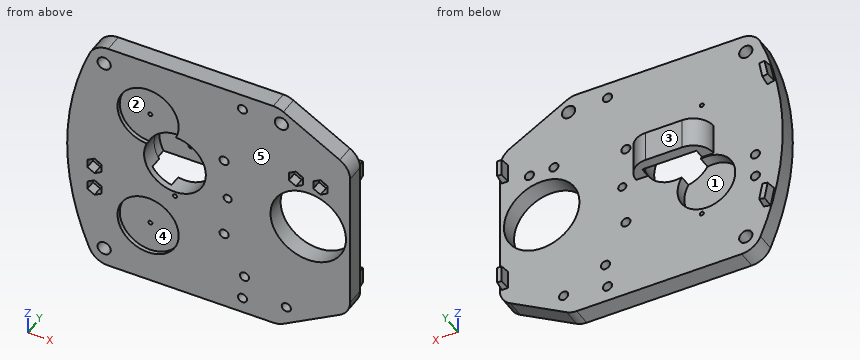
```python
from build123d import *

# Parameters (mm, degrees)
SKETCH1_W                         = 125
SKETCH1_H                         = 120
TOP_BASE_DEPTH                    = 9
SKETCH5_R                         = 14.15
DRIVE_GEAR_HOLE_DEPTH             = 6
SKETCH28_R                        = 15.15
TWO_STAGE_GEAR_HOLE_DEPTH         = 174.51080658
SKETCH8_R                         = 18.5
XL320_FINGER_KNUCKLE_MOUNT_DEPTH  = 174.51080658
SKETCH26_R                        = 1
STRING_HOLES_DEPTH                = 174.51080658
XL320_MOUNT_HOLES_R               = 2.25
XL320_MOUNT_HOLES_M4_DEPTH        = 174.51080658
AX12_MOUNT_HOLES_R                = 2.25
AX12_MOUNT_HOLES_M4_DEPTH         = 174.51080658
NUTS_M4_DEPTH                     = 5
SKETCH34_R                        = 15
HOLES_FOR_M4_IN_FINGER_GEAR_DEPTH = 2
SKETCH31_W                        = 38
SKETCH31_H                        = 15
BOSS_EXTRUDE1_DEPTH               = 10
SKETCH32_R                        = 15.25
CUT_EXTRUDE5_DEPTH                = 5
SKETCH33_R                        = 1
CUT_EXTRUDE6_DEPTH                = 2.5
FILLET2_R                         = 10
CUT_EXTRUDE8_DEPTH                = 174.565549577
FILLET4_R                         = 10
SKETCH37_R                        = 3.25
CONNECT_HOLES_M6_DEPTH            = 10
SKETCH41_R                        = 2
CONNECT_TO_HOUSE_M4_DEPTH         = 174.565549577
SKETCH42_W                        = 3
SKETCH42_H                        = 9
HOUSING_FITS_DEPTH                = 5
HOUSING_FITS_DRAFT                = 5
HOUSING_FITS_PROFILE_2_DEPTH      = 5
HOUSING_FITS_PROFILE_2_DRAFT      = 5
HOUSING_FITS_PROFILE_3_DEPTH      = 5
HOUSING_FITS_PROFILE_3_DRAFT      = 5
HOUSING_FITS_PROFILE_4_DEPTH      = 5
HOUSING_FITS_PROFILE_4_DRAFT      = 5
SKETCH43_R                        = 1
M2_SHAFT_HOLE_DEPTH               = 2


with BuildPart() as part:
    # Sketch1 → Top_Base (new body)
    with BuildSketch(Plane(origin=(0, 0, 0), x_dir=(1, 0, 0), z_dir=(0, 1, 0))):
        with BuildLine():
            ThreePointArc((0, 120), (-13.654246239, 60), (0, 0))
            Line((0, 0), (0, 120))
        make_face()
        with Locations((62.5, 60)):
            Rectangle(SKETCH1_W, SKETCH1_H)
    extrude(amount=TOP_BASE_DEPTH)

    # Sketch5 → Drive_Gear_Hole (cut)
    with BuildSketch(Plane(origin=(0, 9, 0), x_dir=(1, 0, 0), z_dir=(0, 1, 0))):
        with Locations(Location((23.75, 73.41386581, 0), (0, 0, 270))):
            Circle(SKETCH5_R)
    extrude(amount=-DRIVE_GEAR_HOLE_DEPTH, mode=Mode.SUBTRACT)

    # Sketch28 → Two_Stage_Gear_Hole (cut, through all)
    with BuildSketch(Plane(origin=(0, 9, 0), x_dir=(1, 0, 0), z_dir=(0, 1, 0))):
        with Locations(Location((39.169567191, 51.25, 0), (0, 0, 270))):
            Circle(SKETCH28_R)
    extrude(amount=-TWO_STAGE_GEAR_HOLE_DEPTH, mode=Mode.SUBTRACT)

    # Sketch8 → XL320_Finger_Knuckle_Mount (cut, through all)
    with BuildSketch(Plane(origin=(0, 9, 0), x_dir=(1, 0, 0), z_dir=(0, 1, 0))):
        with Locations(Location((104.5, 60, 0), (0, 0, 270))):
            Circle(SKETCH8_R)
    extrude(amount=-XL320_FINGER_KNUCKLE_MOUNT_DEPTH, mode=Mode.SUBTRACT)

    # Sketch26 → String_Holes (cut, through all)
    with BuildSketch(Plane.XZ.offset(-9)):
        with Locations(Location((26, -30, 0), (0, 0, 270))):
            Circle(SKETCH26_R)
        with Locations(Location((26, -90, 0), (0, 0, 90))):
            Circle(SKETCH26_R)
    extrude(amount=STRING_HOLES_DEPTH, mode=Mode.SUBTRACT)

    # XL320_Mount_Holes → XL320_Mount_Holes_(M4) (cut, through all)
    with BuildSketch(Plane(origin=(0, 9, 0), x_dir=(1, 0, 0), z_dir=(0, 1, 0))):
        with Locations(Location((110.5, 36, 0), (0, 0, 270))):
            Circle(XL320_MOUNT_HOLES_R)
        with Locations(Location((98.5, 36, 0), (0, 0, 270))):
            Circle(XL320_MOUNT_HOLES_R)
        with Locations(Location((-0.25, 79.41386581, 0), (0, 0, 270))):
            Circle(XL320_MOUNT_HOLES_R)
        with Locations(Location((-0.25, 67.41386581, 0), (0, 0, 270))):
            Circle(XL320_MOUNT_HOLES_R)
    extrude(amount=-XL320_MOUNT_HOLES_M4_DEPTH, mode=Mode.SUBTRACT)

    # AX12_Mount_Holes → AX12_Mount_Holes_(M4) (cut, through all)
    with BuildSketch(Plane(origin=(0, 9, 0), x_dir=(1, 0, 0), z_dir=(0, 1, 0))):
        with Locations(Location((72.25, 112.25, 0), (0, 0, 270))):
            Circle(AX12_MOUNT_HOLES_R)
        with Locations(Location((63.25, 80.25, 0), (0, 0, 270))):
            Circle(AX12_MOUNT_HOLES_R)
        with Locations(Location((73.25, 100, 0), (0, 0, 270))):
            Circle(AX12_MOUNT_HOLES_R)
        with Locations(Location((93.75, 109, 0), (0, 0, 270))):
            Circle(AX12_MOUNT_HOLES_R)
        with Locations(Location((63.25, 39.75, 0), (0, 0, 270))):
            Circle(AX12_MOUNT_HOLES_R)
        with Locations(Location((72.25, 7.75, 0), (0, 0, 270))):
            Circle(AX12_MOUNT_HOLES_R)
    extrude(amount=-AX12_MOUNT_HOLES_M4_DEPTH, mode=Mode.SUBTRACT)

    # Sketch27 → Nuts_(M4) (cut)
    with BuildSketch(Plane.XZ):
        Polygon((110.5, -31.958548116), (107, -33.979274058), (107, -38.020725942), (110.5, -40.041451884), (114, -38.020725942), (114, -33.979274058), align=None)
        Polygon((98.5, -31.958548116), (95, -33.979274058), (95, -38.020725942), (98.5, -40.041451884), (102, -38.020725942), (102, -33.979274058), align=None)
        Polygon((3.25, -65.393139868), (-0.25, -63.372413926), (-3.75, -65.393139868), (-3.75, -69.434591752), (-0.25, -71.455317694), (3.25, -69.434591752), align=None)
        Polygon((-3.75, -77.393139868), (-3.75, -81.434591752), (-0.25, -83.455317694), (3.25, -81.434591752), (3.25, -77.393139868), (-0.25, -75.372413926), align=None)
    extrude(amount=-NUTS_M4_DEPTH, mode=Mode.SUBTRACT)

    # Sketch34 → Holes_For_M4_In_Finger_Gear (cut)
    with BuildSketch(Plane.XZ):
        with Locations((26, -30)):
            Circle(SKETCH34_R)
        with Locations(Location((26, -90, 0), (0, 0, 270))):
            Circle(SKETCH34_R)
    extrude(amount=-HOLES_FOR_M4_IN_FINGER_GEAR_DEPTH, mode=Mode.SUBTRACT)

    # Sketch31 → Boss-Extrude1 (add)
    with BuildSketch(Plane(origin=(0, 9, 0), x_dir=(1, 0, 0), z_dir=(0, 1, 0))):
        with Locations((39.169567191, 51.25)):
            Rectangle(SKETCH31_W, SKETCH31_H)
    extrude(amount=BOSS_EXTRUDE1_DEPTH)

    # Sketch32 → Cut-Extrude5 (cut)
    with BuildSketch(Plane.XZ.offset(-9)):
        with Locations((39.169567191, -51.25)):
            Circle(SKETCH32_R)
    extrude(amount=-CUT_EXTRUDE5_DEPTH, mode=Mode.SUBTRACT)

    # Sketch33 → Cut-Extrude6 (cut)
    with BuildSketch(Plane.XZ.offset(-14)):
        with Locations(Location((39.169567191, -51.25, 0), (0, 0, 270))):
            Circle(SKETCH33_R)
    extrude(amount=-CUT_EXTRUDE6_DEPTH, mode=Mode.SUBTRACT)

    # Fillet2
    fillet2_edges = [part.edges().sort_by_distance(p)[0] for p in [
        (58.169567191, 19, -51.25),
        (20.169567191, 19, -51.25),
    ]]
    fillet(fillet2_edges, radius=FILLET2_R - 0.0001)  # a hair under: the kernel refuses the full size

    # Sketch36 → Cut-Extrude8 (cut, through all)
    with BuildSketch(Plane(origin=(0, 9, 0), x_dir=(1, 0, 0), z_dir=(0, 1, 0))):
        Polygon((90, 120), (125, 100), (125, 120), align=None)
        Polygon((125, 0), (90, 0), (125, 20), align=None)
    extrude(amount=-CUT_EXTRUDE8_DEPTH, mode=Mode.SUBTRACT)

    # Fillet4
    fillet4_edges = [part.edges().sort_by_distance(p)[0] for p in [
        (90, 4.5, -120),
        (125, 4.5, -100),
        (125, 4.5, -20),
        (90, 4.5, 0),
        (0, 4.5, -120),
        (0, 4.5, 0),
    ]]
    fillet(fillet4_edges, radius=FILLET4_R)

    # Sketch37 → Connect_Holes_(M6) (cut)
    with BuildSketch(Plane(origin=(0, 9, 0), x_dir=(1, 0, 0), z_dir=(0, 1, 0))):
        with Locations(Location((4.459226107, 111.152938298, 0), (0, 0, 270))):
            Circle(SKETCH37_R)
        with Locations(Location((4.459226107, 8.847061702, 0), (0, 0, 270))):
            Circle(SKETCH37_R)
        with Locations(Location((91.344355629, 8.205555711, 0), (0, 0, 270))):
            Circle(SKETCH37_R)
    extrude(amount=-CONNECT_HOLES_M6_DEPTH, mode=Mode.SUBTRACT)

    # Sketch41 → Connect_To_House_(M4) (cut, through all)
    with BuildSketch(Plane(origin=(0, 9, 0), x_dir=(1, 0, 0), z_dir=(0, 1, 0))):
        with Locations(Location((65, 60, 0), (0, 0, 270))):
            Circle(SKETCH41_R)
    extrude(amount=-CONNECT_TO_HOUSE_M4_DEPTH, mode=Mode.SUBTRACT)


with BuildPart() as housing_fits_tool:
    # Sketch42 → Housing_Fits (with draft: the straight prism first)
    with BuildSketch(Plane(origin=(0, 9, 0), x_dir=(1, 0, 0), z_dir=(0, 1, 0))):
        with Locations((122.5, 30.5)):
            Rectangle(SKETCH42_W, SKETCH42_H)
    extrude(amount=HOUSING_FITS_DEPTH)
    # Housing_Fits: the draft: its side faces are tilted about the plane it starts from
    housing_fits_sides = [housing_fits_tool.faces().sort_by_distance(p)[0] for p in [
        (124, 11.5, -30.5),
        (122.5, 11.5, -35),
        (121, 11.5, -30.5),
        (122.5, 11.5, -26),
    ]]
    draft(housing_fits_sides, Plane(origin=(0, 9, 0), x_dir=(1, 0, 0), z_dir=(0, 1, 0)), HOUSING_FITS_DRAFT)


with BuildPart() as part_1:
    add(part.part)

    # Housing_Fits: add housing_fits_tool
    add(housing_fits_tool.part)


with BuildPart() as housing_fits_profile_2_tool:
    # Sketch42 → Housing_Fits profile 2 (with draft: the straight prism first)
    with BuildSketch(Plane(origin=(0, 9, 0), x_dir=(1, 0, 0), z_dir=(0, 1, 0))):
        Polygon((-9.533377338, 30.232888291), (-7.782151246, 21.404909633), (-4.349048435, 22.085942002), (-6.100274527, 30.91392066), align=None)
    extrude(amount=HOUSING_FITS_PROFILE_2_DEPTH)
    # Housing_Fits profile 2: the draft: its side faces are tilted about the plane it starts from
    housing_fits_profile_2_sides = [housing_fits_profile_2_tool.faces().sort_by_distance(p)[0] for p in [
        (-8.657764292, 11.5, -25.818898962),
        (-6.065599841, 11.5, -21.745425818),
        (-5.224661481, 11.5, -26.499931331),
        (-7.816825933, 11.5, -30.573404475),
    ]]
    draft(housing_fits_profile_2_sides, Plane(origin=(0, 9, 0), x_dir=(1, 0, 0), z_dir=(0, 1, 0)), HOUSING_FITS_PROFILE_2_DRAFT)


with BuildPart() as part_2:
    add(part_1.part)

    # Housing_Fits profile 2: add housing_fits_profile_2_tool
    add(housing_fits_profile_2_tool.part)


with BuildPart() as housing_fits_profile_3_tool:
    # Sketch42 → Housing_Fits profile 3 (with draft: the straight prism first)
    with BuildSketch(Plane(origin=(0, 9, 0), x_dir=(1, 0, 0), z_dir=(0, 1, 0))):
        Polygon((-4.349048435, 97.914057998), (-7.782151246, 98.595090367), (-9.533377338, 89.767111709), (-6.100274527, 89.08607934), align=None)
    extrude(amount=HOUSING_FITS_PROFILE_3_DEPTH)
    # Housing_Fits profile 3: the draft: its side faces are tilted about the plane it starts from
    housing_fits_profile_3_sides = [housing_fits_profile_3_tool.faces().sort_by_distance(p)[0] for p in [
        (-6.065599841, 11.5, -98.254574182),
        (-8.657764292, 11.5, -94.181101038),
        (-7.816825933, 11.5, -89.426595525),
        (-5.224661481, 11.5, -93.500068669),
    ]]
    draft(housing_fits_profile_3_sides, Plane(origin=(0, 9, 0), x_dir=(1, 0, 0), z_dir=(0, 1, 0)), HOUSING_FITS_PROFILE_3_DRAFT)


with BuildPart() as part_3:
    add(part_2.part)

    # Housing_Fits profile 3: add housing_fits_profile_3_tool
    add(housing_fits_profile_3_tool.part)


with BuildPart() as housing_fits_profile_4_tool:
    # Sketch42 → Housing_Fits profile 4 (with draft: the straight prism first)
    with BuildSketch(Plane(origin=(0, 9, 0), x_dir=(1, 0, 0), z_dir=(0, 1, 0))):
        with Locations((122.5, 89.5)):
            Rectangle(SKETCH42_W, SKETCH42_H)
    extrude(amount=HOUSING_FITS_PROFILE_4_DEPTH)
    # Housing_Fits profile 4: the draft: its side faces are tilted about the plane it starts from
    housing_fits_profile_4_sides = [housing_fits_profile_4_tool.faces().sort_by_distance(p)[0] for p in [
        (122.5, 11.5, -94),
        (121, 11.5, -89.5),
        (122.5, 11.5, -85),
        (124, 11.5, -89.5),
    ]]
    draft(housing_fits_profile_4_sides, Plane(origin=(0, 9, 0), x_dir=(1, 0, 0), z_dir=(0, 1, 0)), HOUSING_FITS_PROFILE_4_DRAFT)


with BuildPart() as part_4:
    add(part_3.part)

    # Housing_Fits profile 4: add housing_fits_profile_4_tool
    add(housing_fits_profile_4_tool.part)

    # Sketch43 → M2_Shaft_Hole (cut)
    with BuildSketch(Plane.XZ):
        with Locations(Location((39.169567191, -68.75, 0), (0, 0, 270))):
            Circle(SKETCH43_R)
    extrude(amount=-M2_SHAFT_HOLE_DEPTH, mode=Mode.SUBTRACT)


solid = part_4.part
```
The model under review builds one solid part; all positions refer to its coordinate system, in mm. Face numbers are marked on the shaded views. A direction names the side the tool comes from. Round coordinates to 2 decimals unless told otherwise and drop trailing zeros. Answer as a JSON object with one key per item and string values. Group by question number.
1) Mouldability with a two-part tool opening along Z and no side actions: class the marked faces 4 and 5 as released by +Z, released by -Z, zero draft, split by the parting line, or undercut.
2) For the marked faces 1, 2 and 3, list the 3-axis set-ups (+Z, -Z, +X, -X, +Y, -Y) from which the entire face can be reached by the end or side of a thin tool; tool diameter is ignored.
3) For pin 1 Ø1.2 at (x, z) = (-6.5, -95.5) entering from +Y; pin 2 Ø3.5 at (x, z) = (63.25, -39.75) entering from -Y; pin 3 Ø11 at (x, y) = (47.5, 15) entering from -Z; pin 4 Ø1.5 at (y, z) = (5.5, -14.5) entering from -X, all flat-tipped, find the tip position at first contact; note any pin that passes through.
4) For line 1 (Z direction, x = 0, y = 3.75); line 2 (Z direction, x = 1, y = 8.25); line 3 (Z direction, x = 26, y = 7), list the stretches that pass through material, from the lowest coordinate up. Write a range as [from, to].
Result set:
{
 "1": {"face 4": "undercut", "face 5": "zero draft"},
 "2": {"face 1": "+Y", "face 2": "-Y", "face 3": "+Z, -Z, +X, -X, +Y"},
 "3": {"pin 1": "y = 14", "pin 2": "through", "pin 3": "z = -58.75", "pin 4": "x = -6.23"},
 "4": {"line 1": "[-117.63, -83.31], [-75.52, -71.31], [-63.52, -2.37]", "line 2": "[-118.38, -81.28], [-77.54, -69.28], [-65.54, -1.62]", "line 3": "[-120, -91], [-89, -87.38], [-59.44, -58.74], [-43.76, -31], [-29, 0]"}
}
